Read the model definition and answer for the solid it produces. Units are mm, in the model's axes. Coordinates: 2 decimals unless noted, no trailing zeros. Order: outer loops, then holes, each group sorted by start corner. A loop starts at its lowest first (then second) coordinate and runs counter-clockwise, first axis right, second up. Notation, with made-up numbers: (-14, 34.5) -> (-10, 34.5) arc R26 ccw to (-10, 56.5) -> close; hole circle Ø9 at (-9, 7). An arc over 180 degrees is marked (long way). Answer as a JSON object with one key per item and string values. Group by question number.
1) Section A-A on x = -100 is taken. Determine the outline of the cut face in (y, z).
2) Section B-B on y = -50 is taken. Determine the outline of the cut face in (x, z).
3) Determine the mould class of faces 1 (the flat face through (-101, -27, 0)), 2 (the cylindrical face through (-119.98, -49.12, 1.48)) for opening direction X: released by +X, released by -X, zero draft, split by the parting line, or undercut.
4) Consider L1, parallel to Y at x = -100, z = 1; L2, parallel to X at y = -22, z = 1.45; L3, parallel to X at y = -65, z = 1.05. Determine where each line is inside the solid, lowest interval first.
5) Section C-C on x = -132 is taken. Determine the outline of the cut face in (y, z).
6) Given pin 1 (24 mm diameter, centred on x = -100, y = -50, fed in from +Z); pin 2 (0.9 mm diameter, centred on y = -98, z = 1, fed in from +X); pin 3 (1.5 mm diameter, centred on y = -31.5, z = 1.5, fed in from +X), each flat-ended and moving along its own axis, determine where each tip first touches the part or whether it passes through.
from build123d import *

# Parameters (mm, degrees)
F0_R     = 20
F1_DEPTH = 3


with BuildPart() as f1:
    # F0 (on Top) → F1 (new body)
    with BuildSketch(Plane.XY):
        Polygon((0, -20), (0, 0), (-40, 0), (-40, -3), (-80, -3), (-80, 0), (-120, 0), (-120, -3), (-160, -3), (-160, 0), (-200, 0), (-200, -20), (-197, -20), (-197, -40), (-200, -40), (-200, -60), (-197, -60), (-197, -80), (-200, -80), (-200, -100), (-160, -100), (-160, -97), (-120, -97), (-120, -100), (-80, -100), (-80, -97), (-40, -97), (-40, -100), (0, -100), (0, -80), (-3, -80), (-3, -60), (0, -60), (0, -40), (-3, -40), (-3, -20), align=None)
        with Locations((-100, -50)):
            Circle(F0_R, mode=Mode.SUBTRACT)
    extrude(amount=F1_DEPTH)


solid = f1.part
Worked answers:
{
 "1": {"outline": "(-100, 0) -> (-70, 0) -> (-70, 3) -> (-100, 3) -> close; (-30, 0) -> (0, 0) -> (0, 3) -> (-30, 3) -> close"},
 "2": {"outline": "(-200, 0) -> (-120, 0) -> (-120, 3) -> (-200, 3) -> close; (-80, 0) -> (0, 0) -> (0, 3) -> (-80, 3) -> close"},
 "3": {"face 1": "zero draft", "face 2": "undercut"},
 "4": {"L1": "y = -100 to -70, -30 to 0", "L2": "x = -197 to -3", "L3": "x = -197 to -113.23, -86.77 to -3"},
 "5": {"outline": "(-97, 0) -> (-3, 0) -> (-3, 3) -> (-97, 3) -> close"},
 "6": {"pin 1": "passes through", "pin 2": "stops at x = 0", "pin 3": "stops at x = -3"}
}
